Check sheet for the modelled part. Datum: model origin and axes. Units: mm. Face numbers are marked on the shaded views. A direction names the side the tool comes from. Coordinates: 2 decimals unless noted, no trailing zeros. Order: outer loops, then holes, each group sorted by start corner. A loop starts at its lowest first (then second) coordinate and runs counter-clockwise, first axis right, second up.
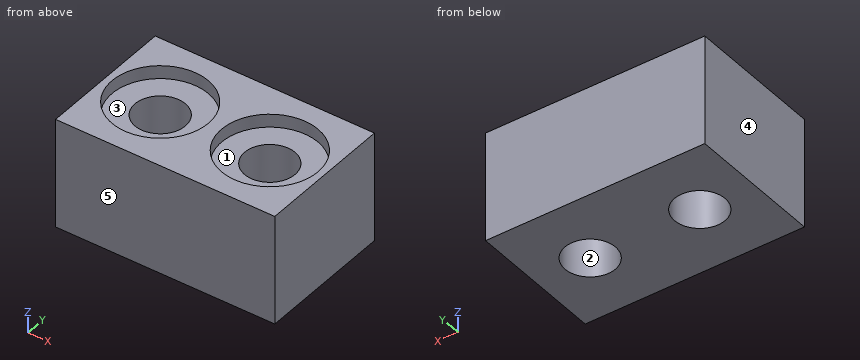
from build123d import *

# Parameters (mm, degrees)
SKETCH1_W           = 12.7
SKETCH1_H           = 7.9375
BOSS_EXTRUDE1_DEPTH = 6.35
SKETCH2_R           = 2.794
CUT_EXTRUDE1_DEPTH  = 0.762
SKETCH3_R           = 1.4605
CUT_EXTRUDE2_DEPTH  = 16.984982022


with BuildPart() as part:
    # Sketch1 → Boss-Extrude1 (new body)
    with BuildSketch(Plane.XY):
        with Locations((6.35, 3.96875)):
            Rectangle(SKETCH1_W, SKETCH1_H)
    extrude(amount=BOSS_EXTRUDE1_DEPTH)

    # Sketch2 → Cut-Extrude1 (cut)
    with BuildSketch(Plane.XY.offset(6.35)):
        with Locations((3.175, 3.96875)):
            Circle(SKETCH2_R)
        with Locations((9.525, 3.96875)):
            Circle(SKETCH2_R)
    extrude(amount=-CUT_EXTRUDE1_DEPTH, mode=Mode.SUBTRACT)

    # Sketch3 → Cut-Extrude2 (cut, through all)
    with BuildSketch(Plane.XY.offset(5.588)):
        with Locations((3.175, 3.96875)):
            Circle(SKETCH3_R)
        with Locations((9.525, 3.96875)):
            Circle(SKETCH3_R)
    extrude(amount=-CUT_EXTRUDE2_DEPTH, mode=Mode.SUBTRACT)


solid = part.part
(1) Thickness scan on probe 1 along X at (y, z) = (4.75, 1.25); probe 2 along X at (y, z) = (3.75, 1); probe 3 along Z at (x, y) = (2.75, 1.5). Record the ranges inside material, lowest first.
Filled in:
probe 1: x = 0 to 1.94, 4.41 to 8.29, 10.76 to 12.7
probe 2: x = 0 to 1.73, 4.62 to 8.08, 10.97 to 12.7
probe 3: z = 0 to 5.59
(2) Tool access check on the marked faces 1 and 2. Record the directions out of +Z, -Z, +X, -X, +Y, -Y that give a thin tool (end or side, any length) a straight path to the whole face; none if there is none.
Filled in:
face 1: +Z
face 2: +Z, -Z
(3) Release check for a two-part mould opening along X. For the marked faces 3, 4 and 5 record: +X half, -X half, draft (parallel to the pull), parting line (faces both ways), or undercut.
Filled in:
face 3: undercut
face 4: -X half
face 5: draft
(4) Cross-section at B-B (z = 1.25). Enter the section's corners in (x, y) (1 decimal), and give its area (3 significant figures).
Filled in:
outline: (0, 0) - (12.7, 0) - (12.7, 7.9) - (0, 7.9) - close; hole circle Ø2.9 at (3.2, 4); hole circle Ø2.9 at (9.5, 4)
area: 87.4 mm2
(5) Cross-section at A-A (x = 9.25). Enter the section's corners in (y, z).
Filled in:
outline: (0, 0) - (2.53, 0) - (2.53, 5.59) - (1.19, 5.59) - (1.19, 6.35) - (0, 6.35) - close; (5.4, 0) - (7.94, 0) - (7.94, 6.35) - (6.75, 6.35) - (6.75, 5.59) - (5.4, 5.59) - close
(6) Go/stop test with flat-tipped pins: P1, Ø1.5, axis at x = 9.5, z = 2.5, coming from the -Y side; P2, Ø1.8, axis at x = 9.52, y = 3.97, coming from the -Z side. Record where each tip stops, or that it passes through.
Filled in:
P1: stops at y = 0
P2: passes through
(7) Cross-section at C-C (x = 7.75). Enter the section's corners in (y, z).
Filled in:
outline: (0, 0) - (7.94, 0) - (7.94, 6.35) - (6.13, 6.35) - (6.13, 5.59) - (1.81, 5.59) - (1.81, 6.35) - (0, 6.35) - close
(8) Cross-section at D-D (y = 6.25). Enter the section's corners in (x, z).
Filled in:
outline: (0, 0) - (12.7, 0) - (12.7, 6.35) - (11.14, 6.35) - (11.14, 5.59) - (7.91, 5.59) - (7.91, 6.35) - (4.79, 6.35) - (4.79, 5.59) - (1.56, 5.59) - (1.56, 6.35) - (0, 6.35) - close
